Source: CAD feature listing. Evaluate the final solid. Frame: model axes, mm. A direction names the side the tool comes from. Give positions to 0.01 mm unless a question says otherwise; leave off trailing zeros. Order: outer loops, then holes, each group sorted by start corner. A loop starts at its lowest first (then second) coordinate and runs counter-clockwise, first axis right, second up. Notation, with made-up numbers: M -14,-24 L 13,-24 A9 cw 13,-15 Z; hole C -30.75,52 d9. An arc over 180 degrees is marked long. Return JSON: item names as keys, results as strings.
from build123d import *

# Parameters (mm, degrees)
BOSS_EXTRUDE1_DEPTH          = 66.675
FILLET1_R                    = 3.175
CUT_EXTRUDE1_DEPTH           = 84.460840368
F_10_0_1935_DIAMETER_HOLE1_D = 4.9149


with BuildPart() as part:
    # Sketch1 → Boss-Extrude1 (new, symmetric)
    with BuildSketch(Plane(origin=(0, 0, 0), x_dir=(1, 0, 0), z_dir=(0, 1, 0))):
        Polygon((0, 28.575), (0, 0), (41.275, 0), (41.275, 3.175), (3.175, 3.175), (3.175, 28.575), align=None)
    extrude(amount=BOSS_EXTRUDE1_DEPTH, both=True)

    # Fillet1
    fillet1_edges = [part.edges().sort_by_distance(p)[0] for p in [
        (41.275, 0, -3.175),
        (3.175, 0, -28.575),
    ]]
    fillet(fillet1_edges, radius=FILLET1_R - 0.0001)  # a hair under: the kernel refuses the full size

    # Sketch4 → Cut-Extrude1 (cut, through all)
    with BuildSketch(Plane.ZY):
        Polygon((0, -66.675), (-28.575, -38.1), (-28.575, -66.675), align=None)
        Polygon((0, 66.675), (-28.575, 38.1), (-28.575, 66.675), align=None)
    extrude(amount=-CUT_EXTRUDE1_DEPTH, mode=Mode.SUBTRACT)

    # #10 (0.1935) Diameter Hole1 (through all)
    with Locations(Plane(origin=(0, 0, -3.175), x_dir=(-1, 0, 0), z_dir=(0, 0, -1))):
        with Locations((-25.4, -53.092781609), (-12.7, -53.092781609), (-12.7, 54.857218391), (-25.4, 54.857218391)):
            Hole(F_10_0_1935_DIAMETER_HOLE1_D / 2)


solid = part.part
1. Set-up query: faces 1 (the face through (21, 1, -3.175)), 2 (the face through (20, 1, 0)). Return all of +Z, -Z, +X, -X, +Y, -Y with unobstructed straight access to the full face (end or side cutting, diameter ignored); none if empty.
Evaluation:
{"face 1": "-Z, +X, +Y, -Y", "face 2": "+Z, +X, -X, +Y, -Y"}
2. Ray query, probe 1 along Y at (x, z) = (25.4, -1.7) (3 decimals); probe 2 along Y at (x, z) = (12.7, -1.8) (3 decimals); probe 3 along X at (y, z) = (-20.5, -22) (3 decimals). Return the intervals inside material, ascending.
Evaluation:
{"probe 1": "y = -64.975 to -55.55, -50.635 to 52.4, 57.315 to 64.975", "probe 2": "y = -64.875 to -55.55, -50.635 to 52.4, 57.315 to 64.875", "probe 3": "x = 0 to 3.175"}
3. First-contact query: pin 1 (10.5 mm diameter, centred on x = 26, y = 22.5, fed in from -Z) (3 decimals); pin 2 (1 mm diameter, centred on y = -4.5, z = -9.5, fed in from +X) (3 decimals); pin 3 (1 mm diameter, centred on y = 32.5, z = -22, fed in from -X). Flat tips, straight axial feed; report the tip coordinate or a pass-through.
Evaluation:
{"pin 1": "stops at z = -3.175", "pin 2": "stops at x = 3.175", "pin 3": "stops at x = 0"}
4. Section query D-D (z = -9.5). Return loops of the section in (x, y) (3 decimals).
Evaluation:
{"outline": "M 0,-57.175 L 3.175,-57.175 L 3.175,57.175 L 0,57.175 Z"}
5. Section query A-A (x = 12.7). Return loops of the section in (y, z) (3 decimals), then the cut area to 3 significant figures.
Evaluation:
{"outline": "M -66.675,0 L -63.5,-3.175 L -55.55,-3.175 L -55.55,0 Z; M -50.635,-3.175 L 52.4,-3.175 L 52.4,0 L -50.635,0 Z; M 57.315,-3.175 L 63.5,-3.175 L 66.675,0 L 57.315,0 Z", "area": "382 mm^2"}
6. Draft query along X for faces 3 (the face through (24.9, -55.5, -1.6)), 4 (the face through (0, 1, -14)), 5 (the face through (13.834, 52.677, -1.565)), 6 (the face through (40.32, 0.93, -2.27)). Return one class per face: pulls with the +X half, pulls with the -X half, needs draft (parallel to the pull), parting line crosses it, or undercut.
Evaluation:
{"face 3": "undercut", "face 4": "pulls with the -X half", "face 5": "undercut", "face 6": "pulls with the +X half"}
7. Section query C-C (x = 33.5). Return loops of the section in (y, z) (3 decimals), then the cut area to 3 significant figures.
Evaluation:
{"outline": "M -66.675,0 L -63.5,-3.175 L 63.5,-3.175 L 66.675,0 Z", "area": "413 mm^2"}
